Drawing for the job (mm, zero at the part's lowest x, y, z). A direction names the side the tool comes from. Give positions to 0.01 mm unless a question says otherwise; leave off trailing zeros. Order: outer loops, then holes, each group sorted by start corner. A loop starts at its lowest first (then second) coordinate and runs counter-clockwise, first axis right, second up. Notation, with made-up numbers: (-5, 87) - (52, 87) arc R17 cw to (52, 99) - close; hole circle Ø5 at (-34, -24). An arc over 180 degrees is marked (long way). Use a Markdown table: item, result.
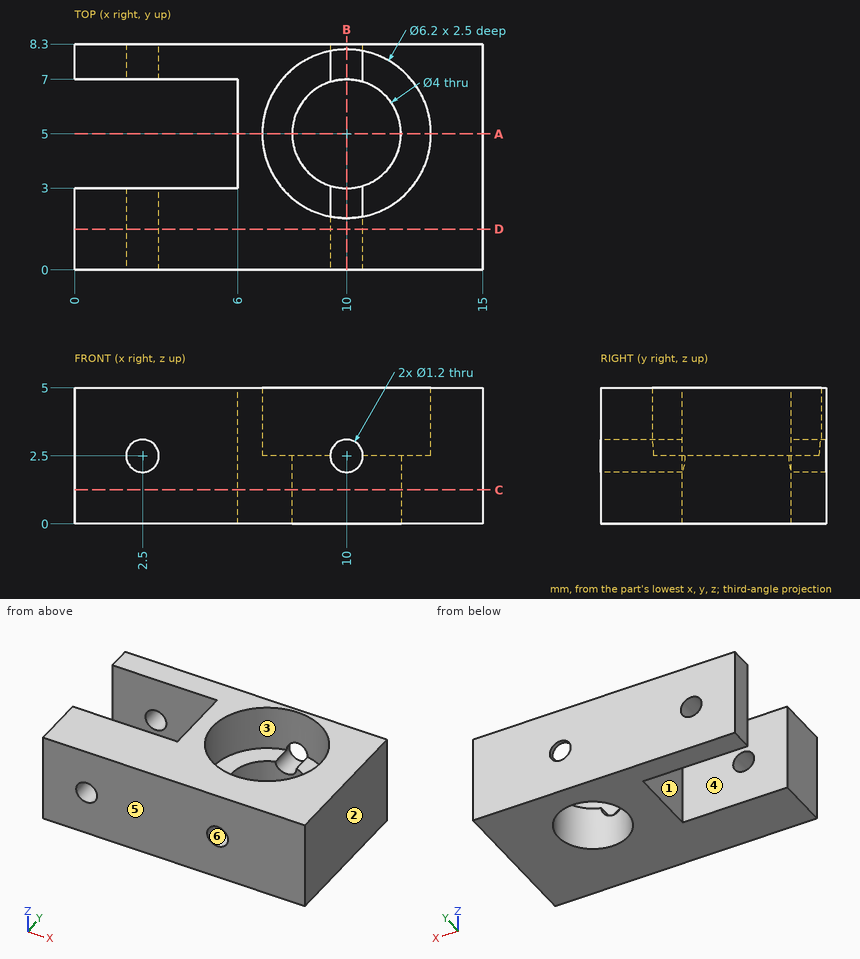
1) Slice it at B-B (x = 10). Write the cut outline in (y, z).
Computed:
| item | result |
|---|---|
| outline | (0, 0) - (3, 0) - (3, 1.9) - (0, 1.9) - close; (0, 3.1) - (1.9, 3.1) - (1.9, 5) - (0, 5) - close; (7, 0) - (8.3, 0) - (8.3, 1.9) - (7, 1.9) - close; (8.1, 3.1) - (8.3, 3.1) - (8.3, 5) - (8.1, 5) - close |
2) Two-plate mould, pull along Y, no slides. Class the marked faces 4, 5 and 6: +Y half, -Y half, draft (parallel to the pull), parting line (faces both ways), or undercut.
Computed:
| item | result |
|---|---|
| face 4 | undercut |
| face 5 | -Y half |
| face 6 | draft |
3) Slice it at D-D (y = 1.5). Write the cut outline in (x, z).
Computed:
| item | result |
|---|---|
| outline | (0, 0) - (15, 0) - (15, 5) - (0, 5) - close; hole circle Ø1.2 at (2.5, 2.5); hole circle Ø1.2 at (10, 2.5) |
4) Slice it at A-A (y = 5). Write the cut outline in (x, z), and give its area (3 significant figures).
Computed:
| item | result |
|---|---|
| outline | (6, 0) - (8, 0) - (8, 2.5) - (6.9, 2.5) - (6.9, 5) - (6, 5) - close; (12, 0) - (15, 0) - (15, 5) - (13.1, 5) - (13.1, 2.5) - (12, 2.5) - close |
| area | 19.5 mm² |
5) Tool access for the marked faces 1, 2 and 3: list every direction of +Z, -Z, +X, -X, +Y, -Y with a clear straight run to the whole face (end or side of a thin tool).
Computed:
| item | result |
|---|---|
| face 1 | +Z, -Z, -X |
| face 2 | +Z, -Z, +X, +Y, -Y |
| face 3 | +Z |
6) Pin check, flat tips, straight feed: P1, Ø1.4, axis at x = 10, z = 2.5, coming from the +Y side; P2, Ø1.3, axis at x = 12, y = 4.5, coming from the +Z side. Stop position of each tip, or through.
Computed:
| item | result |
|---|---|
| P1 | stops at y = 8.3 |
| P2 | stops at z = 2.5 |
7) Slice it at C-C (z = 1.25). Write the cut outline in (x, y).
Computed:
| item | result |
|---|---|
| outline | (0, 0) - (15, 0) - (15, 8.3) - (0, 8.3) - (0, 7) - (6, 7) - (6, 3) - (0, 3) - close; hole circle Ø4 at (10, 5) |
8) Wall check: line 1 (Z direction, x = 10, y = 0.5); line 2 (Y direction, x = 4.5, z = 0.95); line 3 (Z direction, x = 10, y = 7.4). Give the ranges that are in metal, low to high. Write a range as from..to.
Computed:
| item | result |
|---|---|
| line 1 | z = 0..1.9, 3.1..5 |
| line 2 | y = 0..3, 7..8.3 |
| line 3 | z = 0..1.9 |
